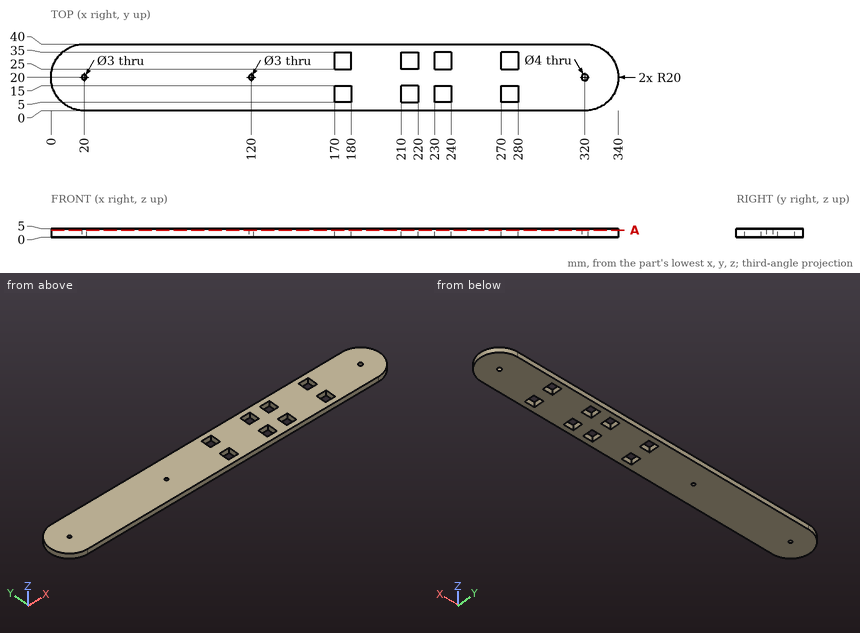
Could you check a few things on this drawing? It's one solid part, dimensions in mm from its lowest x, y, z. Give positions to 0.01 mm unless a question says otherwise; leave off trailing zeros.
1. I need wall thicknesses on L1, parallel to Y at x = 120, z = 2.9; L2, parallel to X at y = 19, z = 3.65; L3, parallel to Y at x = 320, z = 2.75. Which ranges of each line are inside material? Lowest first, please.
Answers below:
L1: y = 0 to 18.5, 21.5 to 40
L2: x = 0.03 to 18.88, 21.12 to 118.88, 121.12 to 318.27, 321.73 to 339.97
L3: y = 0 to 18, 22 to 40
2. Suppose I cut it at A-A (z = 4.15). State how many separate pieces and enclosed holes the cut face has, plus the area to 3 significant figures.
Answers below:
separate pieces: 1
enclosed holes: 11
area: 12,400 mm2
3. For pin 1 (2 mm diameter, centred on y = 31.5, z = 3.5, fed in from +X); pin 2 (3 mm diameter, centred on y = 13.5, z = 2, fed in from -X); pin 3 (2 mm diameter, centred on y = 32, z = 2, fed in from -X), each with a flat end and sliding along its axis, tell me the tip position at first contact or that it passes through.
Answers below:
pin 1: stops at x = 337.02
pin 2: stops at x = 0.64
pin 3: stops at x = 3.3
